The listing builds one solid part. Answer for the finished solid, in the listing's coordinates (mm). Face numbers are marked on the shaded views. A direction names the side the tool comes from. Give positions to 0.01 mm unless a question says otherwise; leave off trailing zeros. Write each loop counter-clockwise with the first axis right and the second up, starting at its lowest first coordinate (ties: lowest second). Pieces come first, ordered by that corner, then holes. Notation, with made-up numbers: (73.5, -7) -> (82.5, -7) arc R24 cw to (82.5, 31) -> close; hole circle Ø10 at (-6, 49). An arc over 180 degrees is marked (long way). Write each question's results on one line, items separated by ' | '. Start each with the question number.
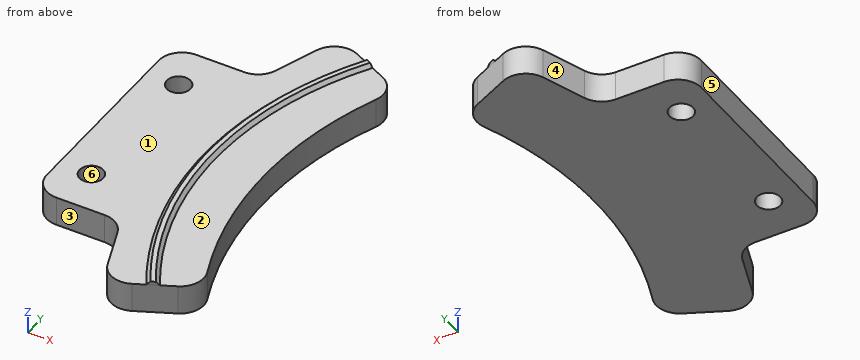
from build123d import *

# Parameters (mm, degrees)
F1_DEPTH = 6.35
F3_DEPTH = 0.762
F4_SIZE  = 0.76199
F5_R     = 2.5527
F6_DEPTH = 6.351
F7_R     = 5.08


# Not quite as in the source:
# - a fillet or chamfer is up to 0.001 mm smaller than in the source, because OpenCascade refuses the exact size


with BuildPart() as f1:
    # F0 (on Top) → F1 (new body)
    with BuildSketch(Plane.XY):
        with BuildLine():
            Line((19.05, 25.4), (0, 25.4))
            Line((0, 25.4), (0, -25.4))
            Line((0, -25.4), (19.05, -25.4))
            Line((19.05, -25.4), (25.5654837304, -43.301144426))
            Line((25.5654837304, -43.301144426), (42.7578812746, -35.0960261037))
            ThreePointArc((42.7578812746, -35.0960261037), (34.8122963703, 0), (42.7578812746, 35.0960261037))
            Line((42.7578812746, 35.0960261037), (25.5654837304, 43.301144426))
            Line((25.5654837304, 43.301144426), (19.05, 25.4))
        make_face()
    extrude(amount=F1_DEPTH)

    # F2 (on face) → F3 (join)
    with BuildSketch(Plane.XY.offset(6.35)):
        with BuildLine():
            Line((35.3141257953, 38.64857858), (33.0094497647, 39.7484914617))
            ThreePointArc((33.0094497647, 39.7484914617), (21.8558198534, 0), (33.0094497647, -39.7484914617))
            Line((33.0094497647, -39.7484914617), (35.3141257953, -38.64857858))
            ThreePointArc((35.3141257953, -38.64857858), (24.3958198534, 0), (35.3141257953, 38.64857858))
        make_face()
    extrude(amount=F3_DEPTH)

    # F4 (size 0.762 in the source; OpenCascade refuses exactly that, so slightly less here)
    f4_edges = [f1.edges().sort_by_distance(p)[0] for p in [
        (21.85582, 0, 7.112),
        (24.39582, 0, 7.112),
    ]]
    chamfer(f4_edges, length=F4_SIZE)

    # F5 (on face) → F6 (cut, through all)
    with BuildSketch(Plane.XY.offset(6.35)):
        with Locations((6.985, 15.875)):
            Circle(F5_R)
        with Locations((6.985, -15.875)):
            Circle(F5_R)
    extrude(amount=-F6_DEPTH, mode=Mode.SUBTRACT)

    # F7
    f7_edges = [f1.edges().sort_by_distance(p)[0] for p in [
        (0, -25.4, 3.175),
        (19.05, -25.4, 3.175),
        (25.565484, -43.301144, 3.175),
        (42.757881, -35.096026, 3.175),
        (0, 25.4, 3.175),
        (19.05, 25.4, 3.175),
        (25.565484, 43.301144, 3.175),
        (42.757881, 35.096026, 3.175),
    ]]
    fillet(f7_edges, radius=F7_R)


solid = f1.part
1. Section B-B (x = 11.5) is taken. Write down the section's boundary in (y, z).
2. A tool of negligible diameter and unlimited length cuts with its end or side. For the marked faces 1, 2 and 3, from which of +Z, -Z, +X, -X, +Y, -Y can it reach the whole face along a straight path? Write none if from no direction.
3. Section C-C (x = 19.5) is taken. Write down the section's boundary in (y, z).
4. Section A-A (z = 2.75) is taken. Write down the section's boundary in (x, y) (1 decimal).
5. Each of these flat-tipped pins is pushed along its axis until it touches: pin 1 Ø18.5 at (x, y) = (35.5, 1.5) entering from +Z; pin 2 Ø1.5 at (x, z) = (26.5, 5) entering from -Y; pin 3 Ø2 at (y, z) = (21.5, 1) entering from -X. Where does it stop, or does it pass through?
6. The mould has two halves that part along Y. Classify the marked faces 4, 5 and 6: pulls with the +Y half, pulls with the -Y half, needs draft (parallel to the pull), parting line crosses it, or undercut.
7. Consider probe 1 along Y at (x, z) = (7, 1.25); probe 2 along Y at (x, z) = (6, 1); probe 3 along Z at (x, y) = (28, -9). Determine where each line is inside the solid, lowest interval first. Write a range as [from, to].
Results:
1) outline: (-25.4, 0) -> (25.4, 0) -> (25.4, 6.35) -> (-25.4, 6.35) -> close
2) face 1: +Z, -X | face 2: +Z, +X | face 3: +Z, -Z, -X, -Y
3) outline: (-27.36, 0) -> (27.36, 0) -> (27.36, 6.35) -> (-27.36, 6.35) -> close
4) outline: (0, -20.3) arc R5.1 ccw to (5.1, -25.4) -> (15.5, -25.4) arc R5.1 cw to (20.3, -28.7) -> (23.7, -38) arc R5.1 ccw to (30.6, -40.9) -> (38.3, -37.2) arc R5.1 ccw to (40.8, -30.7) arc R81.5 cw to (40.8, 30.7) arc R5.1 ccw to (38.3, 37.2) -> (30.6, 40.9) arc R5.1 ccw to (23.7, 38) -> (20.3, 28.7) arc R5.1 cw to (15.5, 25.4) -> (5.1, 25.4) arc R5.1 ccw to (0, 20.3) -> close; hole circle Ø5.1 at (7, -15.9); hole circle Ø5.1 at (7, 15.9)
5) pin 1: stops at z = 6.35 | pin 2: stops at y = -41.25 | pin 3: stops at x = 0
6) face 4: pulls with the +Y half | face 5: needs draft | face 6: undercut
7) probe 1: y = [-25.4, -18.43], [-13.32, 13.32], [18.43, 25.4] | probe 2: y = [-25.4, -18.23], [-13.52, 13.52], [18.23, 25.4] | probe 3: z = [0, 6.35]
